Autodesk Inventor part; units mm, degrees
ref_plane "YZ Plane" through (0, 0, 0) normal (1, 0, 0) x (0, 1, 0)
ref_plane "XZ Plane" through (0, 0, 0) normal (0, 1, 0) x (-1, 0, 0)
ref_plane "XY Plane" through (0, 0, 0) normal (0, 0, 1) x (1, 0, 0)
sketch "草圖1" plane through (0, 0, 0) normal (0, 1, 0) x (-1, 0, 0)
  line L0 (-38, 30) -> (38, 30)
  line L1 (38, 30) -> (38, -30)
  line L2 (38, -30) -> (-38, -30)
  line L3 (-38, -30) -> (-38, 30)
  point P0 (0, 0)
  point P1 (0, -30)
  point P2 (38, 0)
  dimension "d0" = 60
  dimension "d1" = 76
extrude "擠出1" add sketch "草圖1" along normal blind 5
sketch "草圖2" plane through (0, 5, 0) normal (0, 1, 0) x (1, 0, 0)
  line L0 (38, 30) -> (-38, 30)
  line L1 (-38, 30) -> (-38, -30)
  line L2 (-38, -30) -> (38, -30)
  line L3 (38, -30) -> (38, 30)
  line L4 (-27, 30) -> (-27, -30)
  line L5 (27, -30) -> (27, 30)
  point P0 (0, 0)
  dimension "d4" = 11
  dimension "d5" = 11
extrude "擠出2" add sketch "草圖2" along normal blind 55 contours L3 L2 L5 L0 | L4 L2 L1 L0
sketch "草圖3" plane through (38, 0, 30) normal (1, 0, 0) x (0, 0, -1)
  line L0 (60, 0) -> (60, 60)
  line L1 (0, 5) -> (60, 5)
  circle A0 centre (40, 30) radius 11.2
  line L2 (10.7467, 49.2158) -> (40, 30)
  point P0 (30, 0)
  dimension "d8" = 22.4
  dimension "d9" = 25
  dimension "d10" = 20
  dimension "d25" = 35
  dimension "d26" = 33.3
sketch "草圖4" plane through (-38, 0, -30) normal (-1, 0, 0) x (0, 0, 1)
  line L0 (0, 0) -> (0, 60)
  line L1 (0, 5) -> (60, 5)
  circle A0 centre (20, 30) radius 11.2
  line L2 (20, 30) -> (49.2533, 49.2158)
  point P0 (30, 0)
  dimension "d13" = 22.4
  dimension "d14" = 25
  dimension "d15" = 20
  dimension "d41" = 35
  dimension "d42" = 33.3
hole "孔1" at (38, 30, -10) direction (-1, 0, 0) diameter 8.5 end through all counterbore diameter 22.3 counterbore depth 8.5
hole "孔2" at (-38, 30, -10) direction (1, 0, 0) diameter 8.5 end through all counterbore diameter 22.3 counterbore depth 8.5
hole "孔4" at (-38, 49.2158, 19.2533) direction (1, 0, 0) diameter 8.5 depth 11 counterbore diameter 12.3 counterbore depth 6
equation "\"d13\" = d8"
equation "\"d14\" = d9"
equation "\"d15\" = d10"
properties part number "Base"
Check sheet for the modelled part. Datum: model origin and axes. Units: mm. A direction names the side the tool comes from. Give positions to 0.01 mm unless a question says otherwise; leave off trailing zeros. Loops run counter-clockwise (first coordinate to the right, second up) from the corner with the lowest first, then second, coordinate; pieces in that order, holes last. Notation, with made-up numbers: M 36.25,-24 L 93.25,-24 A24 cw 93.25,-11 Z; hole C 25,62.5 d4. An arc over 180 degrees is marked long. Use a Markdown table: item, result. Add a question column.
Q1. Scan lines: line 1 along X through (y, z) = (18, 17); line 2 along Y through (x, z) = (-27.75, -10); line 3 along Y through (x, z) = (-34.75, -10). Record each from-to range of solid material in increasing order. Write a range as [from, to].
Q2. Sectioned sample at D-D, the plane y = 7.5. Record the cut outline in (x, z).
Q3. Sectioned sample at A-A, the plane y = 30. Record the cut outline in (x, z), then the cut area to 3 significant figures.
Q4. Sectioned sample at B-B, the plane z = -10. Record the cut outline in (x, y), then the cut area to 3 significant figures.
Q5. Mould release check, pull along Y, two halves, no side actions. Record for faces 1 (the cylindrical face through (-29.465, 47.939, 23.307)), 2 (the flat face through (6, 3, 30)), 3 (the flat face through (1, 0, 0)), 4 (the flat face through (-29.5, 35, -10)): pulls with the +Y half, pulls with the -Y half, needs draft (parallel to the pull), parting line crosses it, or undercut.
Q6. Sectioned sample at C-C, the plane x = 28.5. Record the cut outline in (y, z).
Q7. Tool access check on faces 5 (the flat face through (0, 5, 0)), 6 (the flat face through (29.5, 35, -10)), 7 (the cylindrical face through (-33.69, 18.945, -11.452)). Record the directions out of +Z, -Z, +X, -X, +Y, -Y that give a thin tool (end or side, any length) a straight path to the whole face; none if there is none.
Q8. Go/stop test with flat-tipped pins: pin 1 (6 mm diameter, centred on x = 0.5, z = -23, fed in from +Y); pin 2 (3.5 mm diameter, centred on y = 48, z = 21, fed in from -X); pin 3 (2 mm diameter, centred on y = 38, z = -6, fed in from -X). Record where each tip stops, or that it passes through.
Verdict:
| question | item | result |
|---|---|---|
| 1 | line 1 | [-38, -27], [27, 38] |
| 1 | line 2 | [0, 25.75], [34.25, 60] |
| 1 | line 3 | [0, 18.85], [41.15, 60] |
| 2 | outline | M -38,-30 L -27,-30 L -27,30 L -38,30 Z; M 27,-30 L 38,-30 L 38,30 L 27,30 Z |
| 3 | outline | M -38,-30 L -27,-30 L -27,-14.25 L -29.5,-14.25 L -29.5,-21.15 L -38,-21.15 Z; M -38,1.15 L -29.5,1.15 L -29.5,-5.75 L -27,-5.75 L -27,30 L -38,30 Z; M 27,-30 L 38,-30 L 38,-21.15 L 29.5,-21.15 L 29.5,-14.25 L 27,-14.25 Z; M 27,-5.75 L 29.5,-5.75 L 29.5,1.15 L 38,1.15 L 38,30 L 27,30 Z |
| 3 | area | 898 mm^2 |
| 4 | outline | M -38,0 L 38,0 L 38,18.85 L 29.5,18.85 L 29.5,25.75 L 27,25.75 L 27,5 L -27,5 L -27,25.75 L -29.5,25.75 L -29.5,18.85 L -38,18.85 Z; M -38,41.15 L -29.5,41.15 L -29.5,34.25 L -27,34.25 L -27,60 L -38,60 Z; M 27,34.25 L 29.5,34.25 L 29.5,41.15 L 38,41.15 L 38,60 L 27,60 Z |
| 4 | area | 1,170 mm^2 |
| 5 | face 1 | undercut |
| 5 | face 2 | needs draft |
| 5 | face 3 | pulls with the -Y half |
| 5 | face 4 | undercut |
| 6 | outline | M 0,-30 L 60,-30 L 60,30 L 0,30 Z; hole C 30,-10 d8.5 |
| 7 | face 5 | +Z, -Z, +Y |
| 7 | face 6 | +X |
| 7 | face 7 | -X |
| 8 | pin 1 | y = 5 |
| 8 | pin 2 | x = 27 |
| 8 | pin 3 | x = -29.5 |
